Part print with two shaded views. Sizes in mm from the minimum x, y, z corner. Give positions to 0.01 mm unless a question says otherwise; leave off trailing zeros. Write each loop counter-clockwise with the first axis right and the second up, starting at its lowest first coordinate (ties: lowest second). Pieces come first, ordered by that corner, then holes. Notation, with made-up numbers: (19, -37) -> (34, -37) arc R27 cw to (34, -19) -> close; hole circle Ø1 at (-27, 66.25). An arc over 180 degrees is marked (long way). Answer as a JSON object with one key per item and string values.
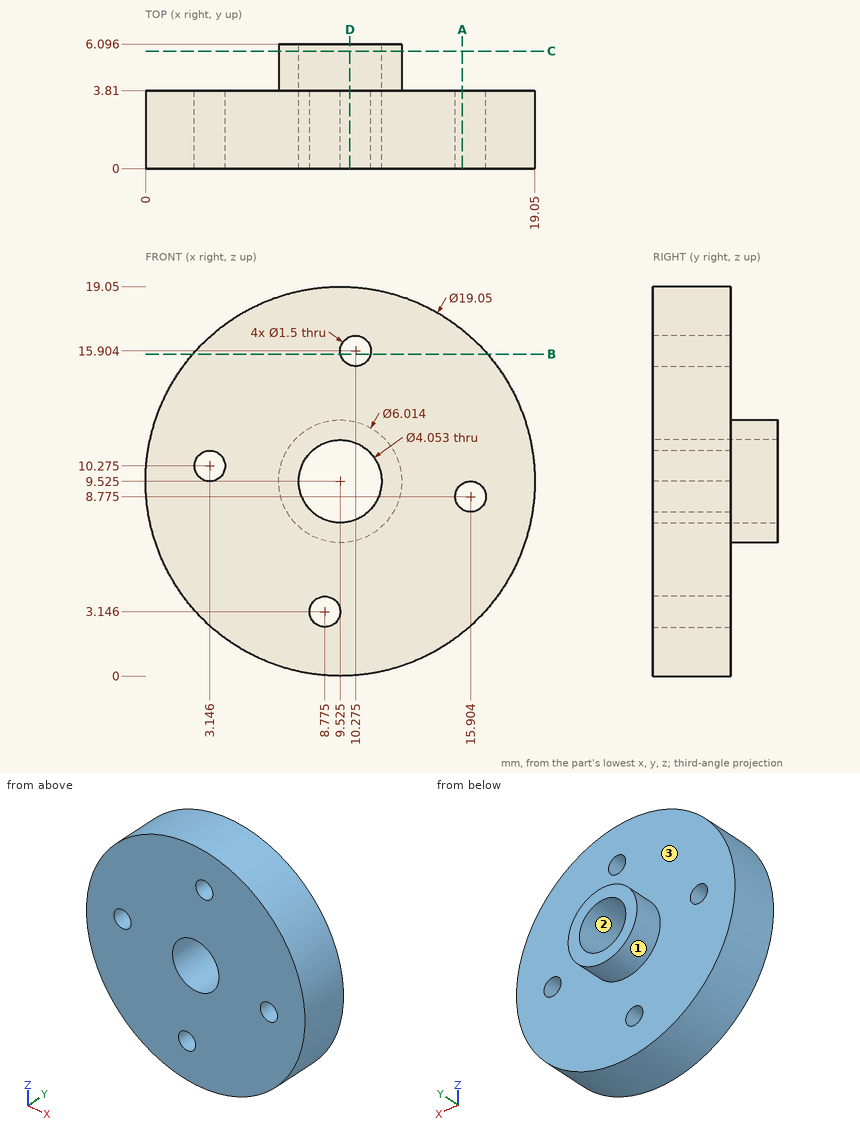
1) Slice it at A-A (x = 15.5). List the corners of the cut face in (y, z).
Model answer:
{"outline": "(0, 2.11) -> (3.81, 2.11) -> (3.81, 8.14) -> (0, 8.14) -> close; (0, 9.41) -> (3.81, 9.41) -> (3.81, 16.94) -> (0, 16.94) -> close"}
2) Mould opens along X. For the marked faces 1, 2 and 3 say: released by +X, released by -X, zero draft, split by the parting line, or undercut.
Model answer:
{"face 1": "split by the parting line", "face 2": "undercut", "face 3": "zero draft"}
3) Pin check, flat tips, straight feed: pin 1 (1.3 mm diameter, centred on x = 3.15, z = 10.27, fed in from +Y); pin 2 (5.5 mm diameter, centred on x = 7, z = 5.5, fed in from +Y); pin 3 (3 mm diameter, centred on y = 3, z = 7, fed in from +X); pin 4 (1.5 mm diameter, centred on x = 10, y = 5.5, fed in from -Z). Stop position of each tip, or through.
Model answer:
{"pin 1": "passes through", "pin 2": "stops at y = 6.1", "pin 3": "stops at x = 18.99", "pin 4": "stops at z = 6.52"}
4) Slice it at C-C (y = 5.75). List the corners of the cut face in (x, z) (1 decimal), then the cut area to 3 significant figures.
Model answer:
{"outline": "circle Ø6 at (9.5, 9.5); hole circle Ø4.1 at (9.5, 9.5)", "area": "15.5 mm2"}
5) Slice it at D-D (x = 10). List the corners of the cut face in (y, z) (1 decimal).
Model answer:
{"outline": "(0, 0) -> (3.8, 0) -> (3.8, 6.6) -> (6.1, 6.6) -> (6.1, 7.6) -> (0, 7.6) -> close; (0, 11.5) -> (6.1, 11.5) -> (6.1, 12.5) -> (3.8, 12.5) -> (3.8, 15.2) -> (0, 15.2) -> close; (0, 16.6) -> (3.8, 16.6) -> (3.8, 19) -> (0, 19) -> close"}
6) Slice it at B-B (z = 15.75). List the corners of the cut face in (x, y).
Model answer:
{"outline": "(2.32, 0) -> (9.54, 0) -> (9.54, 3.81) -> (2.32, 3.81) -> close; (11.01, 0) -> (16.73, 0) -> (16.73, 3.81) -> (11.01, 3.81) -> close"}
7) Wall check: probe 1 along X at (y, z) = (3.75, 8.5) (1 decimal); probe 2 along Z at (x, y) = (9, 1) (1 decimal); probe 3 along Y at (x, z) = (11.75, 2.75). Give the ranges that are in metal, low to high.
Model answer:
{"probe 1": "x = 0.1 to 7.8, 11.3 to 15.2, 16.6 to 19", "probe 2": "z = 0 to 2.4, 3.9 to 7.6, 11.5 to 19", "probe 3": "y = 0 to 3.81"}
